```python
from build123d import *

# Parameters (mm, degrees)
SKETCH1_R           = 75
BOSS_EXTRUDE1_DEPTH = 75
SKETCH2_R           = 75
BOSS_EXTRUDE2_DEPTH = 250
SKETCH3_R           = 50
CUT_EXTRUDE1_DEPTH  = 150


with BuildPart() as part:
    # Sketch1 → Boss-Extrude1 (new body, symmetric)
    with BuildSketch(Plane(origin=(0, 0, 0), x_dir=(0, 0, -1), z_dir=(1, 0, 0))):
        Circle(SKETCH1_R)
    extrude(amount=BOSS_EXTRUDE1_DEPTH, both=True)

    # Sketch2 → Boss-Extrude2 (add)
    with BuildSketch(Plane.XY):
        Circle(SKETCH2_R)
    extrude(amount=BOSS_EXTRUDE2_DEPTH)

    # Sketch3 → Cut-Extrude1 (cut)
    with BuildSketch(Plane.XY.offset(250)):
        Circle(SKETCH3_R)
    extrude(amount=-CUT_EXTRUDE1_DEPTH, mode=Mode.SUBTRACT)


solid = part.part
```
Model file for the job. Use its own axes, mm. A direction names the side the tool comes from. Round coordinates to 2 decimals unless told otherwise and drop trailing zeros. Write each loop counter-clockwise with the first axis right and the second up, starting at its lowest first coordinate (ties: lowest second). Pieces come first, ordered by that corner, then holes. Notation, with made-up numbers: (1.5, 58.5) - (19.5, 58.5) arc R12 cw to (19.5, 81.5) - close; hole circle Ø9 at (10.5, 62.5). An arc over 180 degrees is marked (long way). One line per item, written item: value.
(1) Cut at B-B, the plane z = 135. Give the cut face in (x, y).
Values follow:
outline: circle Ø150 at (0, 0); hole circle Ø100 at (0, 0)
(2) Cut at D-D, the plane z = 25. Give the cut face in (x, y).
Values follow:
outline: (-75, -70.71) - (-25, -70.71) arc R75 ccw to (25, -70.71) - (75, -70.71) - (75, 70.71) - (25, 70.71) arc R75 ccw to (-25, 70.71) - (-75, 70.71) - close
(3) Two-plate mould, pull along X, no slides. Class faces 1 (the flat face through (49, -16, 250)), 2 (the cylindrical face through (47.69, 15.02, 176.05)), 3 (the flat face through (-75, 1, 1)): pulls with the +X half, pulls with the -X half, needs draft (parallel to the pull), parting line crosses it, or undercut.
Values follow:
face 1: needs draft
face 2: undercut
face 3: pulls with the -X half
(4) Cut at A-A, the plane y = 31. Give the cut face in (x, z).
Values follow:
outline: (-75, -68.29) - (75, -68.29) - (75, 68.29) - (68.29, 68.29) - (68.29, 250) - (39.23, 250) - (39.23, 100) - (-39.23, 100) - (-39.23, 250) - (-68.29, 250) - (-68.29, 68.29) - (-75, 68.29) - close
(5) 3-axis set-ups, long thin cutter, end or side, ignore diameter. For faces 4 (the flat face through (-1, 1, 100)), 5 (the flat face through (75, 1, 1)), 6 (the cylindrical face through (1.05, 22.528, -71.537)): which of +Z, -Z, +X, -X, +Y, -Y reach the whole face in a straight line?
Values follow:
face 4: +Z
face 5: +Z, -Z, +X, +Y, -Y
face 6: none
(6) Drop flat-ended pins along their axis: P1, Ø12, axis at y = 8.5, z = 108, coming from the -X side; P2, Ø4, axis at x = -41, z = 176.5, coming from the -Y side; P3, Ø4, axis at x = -13, y = -18.5, coming from the -Z side. Give the stop position or say it passes through.
Values follow:
P1: stops at x = -74.96
P2: stops at y = -64.06
P3: stops at z = -73.16
(7) Wall check: probe 1 along Y at (x, z) = (0, 183); probe 2 along Y at (x, z) = (20.5, 135.5); probe 3 along X at (y, z) = (-43, 173.5). Give the ranges that are in metal, low to high.
Values follow:
probe 1: y = -75 to -50, 50 to 75
probe 2: y = -72.14 to -45.6, 45.6 to 72.14
probe 3: x = -61.45 to -25.51, 25.51 to 61.45
(8) Cut at C-C, the plane x = -24. Give the cut face in (y, z), plus the area to 3 significant figures.
Values follow:
outline: (-71.06, 24) arc R75 ccw (long way) to (71.06, 24) - (71.06, 250) - (43.86, 250) - (43.86, 100) - (-43.86, 100) - (-43.86, 250) - (-71.06, 250) - close
area: 31,300 mm²
